from build123d import *

# Parameters (mm, degrees)
VYSUNOUT1_DEPTH = 6.4
SKICA3_R        = 7.315
VYSUNOUT2_DEPTH = 0.6
SKICA4_R        = 5
VYSUNOUT3_DEPTH = 50
ZKOSIT1_SIZE    = 1
ZAOBLIT1_R      = 0.4


with BuildPart() as part:
    # Skica1 → Vysunout1 (new body)
    with BuildSketch(Plane.XY):
        Polygon((8, -4.618802154), (8, 4.618802154), (0, 9.237604307), (-8, 4.618802154), (-8, -4.618802154), (0, -9.237604307), align=None)
    extrude(amount=VYSUNOUT1_DEPTH)

    # Skica2 → Odebrat otočením1 (revolve, cut)
    with BuildSketch(Plane(origin=(0, 0, 0), x_dir=(1, 0, 0), z_dir=(0, 1, 0))):
        Polygon((8, 0), (19.085125168, 0), (19.085125168, -6.4), align=None)
    revolve(axis=Axis((0, 0, 0), (0, 0, 1)), mode=Mode.SUBTRACT)

    # Skica3 → Vysunout2 (add)
    with BuildSketch(Plane.XY.offset(6.4)):
        Circle(SKICA3_R)
    extrude(amount=VYSUNOUT2_DEPTH)

    # Skica4 → Vysunout3 (add)
    with BuildSketch(Plane.XY.offset(7)):
        Circle(SKICA4_R)
    extrude(amount=VYSUNOUT3_DEPTH)

    # Zkosit1
    zkosit1_edges = [part.edges().sort_by_distance(p)[0] for p in [
        (-5, 0, 57),
    ]]
    chamfer(zkosit1_edges, length=ZKOSIT1_SIZE)

    # Zaoblit1
    zaoblit1_edges = [part.edges().sort_by_distance(p)[0] for p in [
        (-5, 0, 7),
    ]]
    fillet(zaoblit1_edges, radius=ZAOBLIT1_R)


solid = part.part
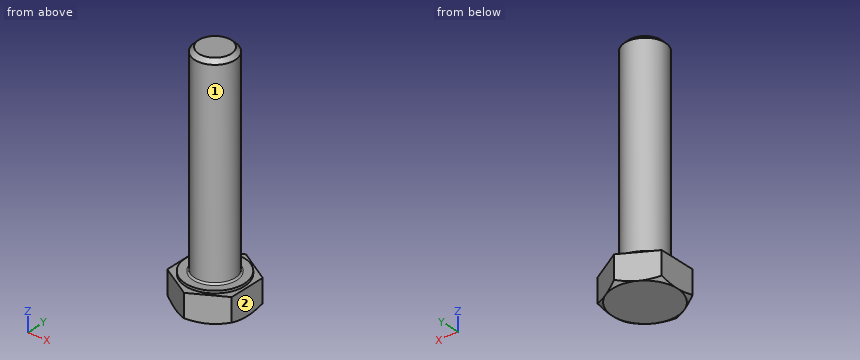
For this review, take the finished solid that the model builds, in its own axes (mm). Face numbers are marked on the shaded views. A direction names the side the tool comes from. Give positions to 0.01 mm unless a question says otherwise; leave off trailing zeros. Order: outer loops, then holes, each group sorted by start corner. A loop starts at its lowest first (then second) coordinate and runs counter-clockwise, first axis right, second up. Notation, with made-up numbers: (-2.5, 4) - (9.5, 4) arc R23 ccw to (9.5, 24) - close; hole circle Ø5 at (-8, 25). An arc over 180 degrees is marked (long way). Answer as a JSON object with one key per item and string values. Group by question number.
Item 1: Machinability: for the marked faces 1 and 2, which of the approach directions +Z, -Z, +X, -X, +Y, -Y give a long, thin tool a straight path to every point of the face, cutting with its end or side? Answer none if there is none.
Item 2: Take a section at A-A on z = 38. Give the boundary of the cut face in (x, y).
Item 3: Clearance check with flat-ended pins moving along their axes: pin 1 Ø1.5 at (x, z) = (3, 21) entering from +Y; pin 2 Ø8 at (x, z) = (6, 50) entering from -Y; pin 3 Ø5 at (y, z) = (-4.5, 29.5) entering from +X. State where each tip first meets the part, or that it passes through.
Item 4: Wall thickness on line 1 along X through (y, z) = (-3, 15); line 2 along Y through (x, z) = (0, 39): over which ranges is each line inside the solid? List them lowest first.
Reported:
{
 "1": {"face 1": "+Z", "face 2": "+Z, -Z, +X, +Y, -Y"},
 "2": {"outline": "circle Ø10 at (0, 0)"},
 "3": {"pin 1": "y = 4.47", "pin 2": "y = -4.58", "pin 3": "x = 4.58"},
 "4": {"line 1": "-4 to 4", "line 2": "-5 to 5"}
}
